```python
from build123d import *


with BuildPart() as part:
    # Esquisse1 → Révolution1 (revolve)
    with BuildSketch(Plane.XY, mode=Mode.PRIVATE) as r_volution1_sk:
        with BuildLine():
            Line((-3.5, 28.9), (-3.4, 29))
            Line((-3.4, 29), (3.4, 29))
            Line((3.4, 29), (3.5, 28.9))
            Line((3.5, 28.9), (3.5, 28.3))
            Line((3.5, 28.3), (3.4, 28.2))
            Line((3.4, 28.2), (0.75, 28.2))
            ThreePointArc((0.75, 28.2), (2.562225595, 25.75), (0.75, 23.3))
            Line((0.75, 23.3), (3.4, 23.3))
            Line((3.4, 23.3), (3.5, 23.2))
            Line((3.5, 23.2), (3.5, 22.6))
            Line((3.5, 22.6), (3.4, 22.5))
            Line((3.4, 22.5), (-3.4, 22.5))
            Line((-3.4, 22.5), (-3.5, 22.6))
            Line((-3.5, 22.6), (-3.5, 23.2))
            Line((-3.5, 23.2), (-3.4, 23.3))
            Line((-3.4, 23.3), (-0.75, 23.3))
            ThreePointArc((-0.75, 23.3), (-2.562225595, 25.75), (-0.75, 28.2))
            Line((-0.75, 28.2), (-3.4, 28.2))
            Line((-3.4, 28.2), (-3.5, 28.3))
            Line((-3.5, 28.3), (-3.5, 28.9))
        make_face()
    revolve(r_volution1_sk.sketch.rotate(Axis((-2.661437812, 0, 0), (1, 0, 0)), 90), axis=Axis((-2.661437812, 0, 0), (1, 0, 0)))


solid = part.part
```
Source: CAD feature listing. Evaluate the final solid. Frame: model axes, mm. Give positions to 0.01 mm unless a question says otherwise; leave off trailing zeros. Loops run counter-clockwise (first coordinate to the right, second up) from the corner with the lowest first, then second, coordinate; pieces in that order, holes last. Notation, with made-up numbers: (-17.5, 62.25) - (41.5, 62.25) arc R20 cw to (41.5, 80.25) - close; hole circle Ø7 at (36.25, 12). An arc over 180 degrees is marked (long way). Use CSV: the item, a comma, the result in double quotes. Start each with the question number.
1. Ray query, L1, parallel to Y at x = 2.2, z = 0; L2, parallel to Y at x = 1.3, z = 0; L3, parallel to Z at x = 1.25, y = 3.5. Return the intervals inside material, ascending.
2. Section A-A (x = -1.5). Output: boundary loops of the cut face in (y, z), then the cut area to 3 significant figures.
3. Draft query along Z for faces 1 (the flat face through (3.5, 5, 22.2)), 2 (the cylindrical face through (0.05, 25.73, 13.38)), 3 (the cylindrical face through (2.09, 20.67, 10.75)). Return one class per face: +Z half, -Z half, draft (parallel to the pull), parting line (faces both ways), or undercut.
4. Pin query (flat end, axial travel): pin 1 (3 mm diameter, centred on x = 1.5, z = -3, fed in from +Y); pin 2 (2 mm diameter, centred on x = 0.5, y = 18, fed in from +Z); pin 3 (1.5 mm diameter, centred on x = -2, y = -13.5, fed in from -Z); pin 4 (3 mm diameter, centred on y = -13.5, z = 15.5, fed in from +X). Return the tip coordinate at first contact, or that it passes through.
Response:
1,L1,"-29 to -28.2, -27.06 to -24.44, -23.3 to -22.5, 22.5 to 23.3, 24.44 to 27.06, 28.2 to 29"
1,L2,"-29 to -28.2, -27.96 to -23.54, -23.3 to -22.5, 22.5 to 23.3, 23.54 to 27.96, 28.2 to 29"
1,L3,"-28.79 to -27.98, -27.77 to -23.25, -23.04 to -22.23, 22.23 to 23.04, 23.25 to 27.77, 27.98 to 28.79"
2,outline,"circle Ø58 at (0, 0); circle Ø55.65 at (0, 0); circle Ø46.6 at (0, 0); hole circle Ø56.4 at (0, 0); hole circle Ø47.35 at (0, 0); hole circle Ø45 at (0, 0)"
2,area,"931 mm²"
3,face 1,"draft"
3,face 2,"parting line"
3,face 3,"undercut"
4,pin 1,"y = 28.96"
4,pin 2,"z = 23.49"
4,pin 3,"z = -26.05"
4,pin 4,"through"
